Here's how the part is built. I have some questions about the finished solid (model axes, mm). A direction names the side the tool comes from. Round coordinates to 2 decimals unless told otherwise and drop trailing zeros. Loops run counter-clockwise (first coordinate to the right, second up) from the corner with the lowest first, then second, coordinate; pieces in that order, holes last. Notation, with made-up numbers: (36, 66) - (76, 66) arc R19 ccw to (76, 81) - close; hole circle Ø5 at (-0.5, -8.5). An arc over 180 degrees is marked (long way). Answer as a JSON object with one key per item and string values. Group by question number.
1) Which directions (+Z, -Z, +X, -X, +Y, -Y) give clear straight access to the entire face, cutting with the end or side of a thin tool? Please do faces 1 (the face through (1, -1, 1)), 2 (the face through (1, 1, 1)).
2) If I drill on line 1 along Y through (x, z) = (-40, -99.3); line 2 along Z through (x, y) = (40, -0.55); line 3 along Z through (x, y) = (-4.5, -2), over which ranges is the centre line in solid material (lowest first)? Write a range as [from, to].
3) I want a section at B-B, the plane x = -8. Please give me the cut outline in (y, z).
4) Will these pins go through, and if not, where does the flat tip stop? P1, Ø3, axis at x = -25, y = -44, coming from the -Z side; P2, Ø5, axis at x = 40, z = -80, coming from the -Y side.
5) I want a section at C-C, the plane z = -6. Please give me the cut outline in (x, y).
6) I want a section at A-A, the plane y = -22.5. Please give me the cut outline in (x, z), then the cut area to 3 significant figures.
7) If we mould it in two halves opening along Z, with no side actions, what happens to faces 3 (the face through (-1, -25, -98)), 4 (the face through (-1, -24, -100)), 5 (the face through (1, -24, 100))? For each: pulls with the +Z half, pulls with the -Z half, needs draft (parallel to the pull), parting line crosses it, or undercut.
Autodesk Inventor part; units mm, degrees
ref_plane "YZ Plane" through (0, 0, 0) normal (1, 0, 0) x (0, 1, 0)
ref_plane "XZ Plane" through (0, 0, 0) normal (0, 1, 0) x (-1, 0, 0)
ref_plane "XY Plane" through (0, 0, 0) normal (0, 0, 1) x (1, 0, 0)
sketch "Skizze1" plane through (0, 0, 0) normal (0, 1, 0) x (-1, 0, 0)
  line L0 (50, -100) -> (-50, -100)
  line L1 (-50, -100) -> (-50, 100)
  line L2 (-50, 100) -> (50, 100)
  line L3 (50, 100) -> (50, -100)
  line L4 (0, -140) -> (0, 140)
  line L5 (70, 0) -> (-70, 0)
  point P0 (0, 0)
  dimension "d0" = 100
  dimension "d1" = 200
extrude "Extrusion1" add sketch "Skizze1" along normal mid plane 2
sketch "Skizze3" plane through (0, -1, 0) normal (0, -1, 0) x (1, 0, 0)
  line L0 (50, -100) -> (-50, -100)
  line L1 (-50, -100) -> (-50, 100)
  line L2 (50, -100) -> (-50, -100)
  line L3 (-50, -100) -> (-50, -98)
  line L4 (-50, -98) -> (50, -98)
  line L5 (50, -98) -> (50, -100)
  line L6 (50, 100) -> (50, -100)
  line L7 (50, 100) -> (-50, 100)
  line L8 (-50, 100) -> (-50, 98)
  line L9 (-50, 98) -> (50, 98)
  line L10 (50, 98) -> (50, 100)
  point P0 (0, 0)
  dimension "d8" = 2
  dimension "d9" = 2
extrude "Extrusion3" add sketch "Skizze3" along normal blind 48 contours L0 L1 L4 L5 | L9 L1 L7 L6
sketch "Skizze4" plane through (-50, 1, 100) normal (0, 0, 1) x (1, 0, 0)
  circle A0 centre (10, -20) radius 1.6
  circle A1 centre (10, -35) radius 1.6
  line L0 (100, -50) -> (0, -50)
  line L1 (0, -50) -> (0, 0)
  point P0 (50, -1)
  dimension "d12" = 3.2
  dimension "d13" = 3.2
  dimension "d14" = 15
  dimension "d15" = 15
  dimension "d16" = 10
  dimension "d17" = 10
extrude "Extrusion4" cut sketch "Skizze4" against normal up to surface (2 mm away)
sketch "Skizze5" plane through (50, 1, -100) normal (0, 0, -1) x (-1, 0, 0)
  circle A0 centre (90, -20) radius 1.6
  circle A1 centre (90, -35) radius 1.6
  line L0 (100, -50) -> (100, 0)
  line L1 (100, -50) -> (0, -50)
  point P0 (50, -1)
  dimension "d20" = 3.2
  dimension "d21" = 3.2
  dimension "d22" = 10
  dimension "d23" = 10
  dimension "d24" = 15
  dimension "d25" = 15
extrude "Extrusion5" cut sketch "Skizze5" against normal up to surface (2 mm away)
sketch "Skizze6" plane through (0, 1, 0) normal (0, 1, 0) x (1, 0, 0)
  line L0 (50, -100) -> (50, 100)
  circle A0 centre (40, -65) radius 1.6
  circle A1 centre (40, -80) radius 1.6
  circle A2 centre (40, 80) radius 1.6
  circle A3 centre (40, 65) radius 1.6
  line L1 (-50, -100) -> (50, -100)
  line L2 (50, 100) -> (-50, 100)
  point P0 (0, 0)
  dimension "d31" = 3.2
  dimension "d32" = 3.2
  dimension "d33" = 3.2
  dimension "d34" = 3.2
  dimension "d35" = 10
  dimension "d36" = 10
  dimension "d37" = 15
  dimension "d38" = 10
  dimension "d39" = 10
  dimension "d40" = 15
  dimension "d41" = 20
  dimension "d42" = 20
extrude "Extrusion6" cut sketch "Skizze6" against normal up to surface (2 mm away)
sketch "Skizze7" plane through (-50, 1, 100) normal (0, 0, 1) x (1, 0, 0)
  circle A0 centre (25, -45) radius 1.6
  line L0 (0, -50) -> (0, 0)
  line L1 (100, -50) -> (0, -50)
  point P0 (50, -1)
  dimension "d45" = 3.2
  dimension "d46" = 25
  dimension "d47" = 5
extrude "Extrusion7" cut sketch "Skizze7" against normal up to surface (2 mm away)
sketch "Skizze8" plane through (50, 1, -100) normal (0, 0, -1) x (-1, 0, 0)
  circle A0 centre (75, -45) radius 1.6
  line L0 (100, -50) -> (100, 0)
  line L1 (100, -50) -> (0, -50)
  point P0 (50, -1)
  dimension "d50" = 3.2
  dimension "d51" = 25
  dimension "d52" = 5
extrude "Extrusion8" cut sketch "Skizze8" against normal up to surface (2 mm away)
properties part number "_3D-Druck"
Outcome:
{
 "1": {"face 1": "+X, -X, -Y", "face 2": "+Z, -Z, +X, -X, +Y"},
 "2": {"line 1": "[-49, -35.6], [-32.4, -20.6], [-17.4, 1]", "line 2": "[-100, -81.6], [-78.4, -66.6], [-63.4, 63.4], [66.6, 78.4], [81.6, 100]", "line 3": "[-100, -98], [98, 100]"},
 "3": {"outline": "(-49, -100) - (1, -100) - (1, 100) - (-49, 100) - (-49, 98) - (-1, 98) - (-1, -98) - (-49, -98) - close"},
 "4": {"P1": "through", "P2": "y = -1"},
 "5": {"outline": "(-50, -1) - (50, -1) - (50, 1) - (-50, 1) - close"},
 "6": {"outline": "(-50, -100) - (50, -100) - (50, -98) - (-50, -98) - close; (-50, 98) - (50, 98) - (50, 100) - (-50, 100) - close", "area": "400 mm^2"},
 "7": {"face 3": "undercut", "face 4": "pulls with the -Z half", "face 5": "pulls with the +Z half"}
}
